Here's the drawing with two shaded views (mm, measured from the low corner). I have some questions. Coordinates: 2 decimals unless noted, no trailing zeros. Loops run counter-clockwise (first coordinate to the right, second up) from the corner with the lowest first, then second, coordinate; pieces in that order, holes last. Notation, with made-up numbers: (3.25, -8) -> (57.25, -8) arc R18 ccw to (57.25, 27) -> close; hole circle Ø11 at (79.25, 28.5). An arc over 180 degrees is marked (long way). Use CSV: the item, a comma, the result in double quotes. Start each with the question number.
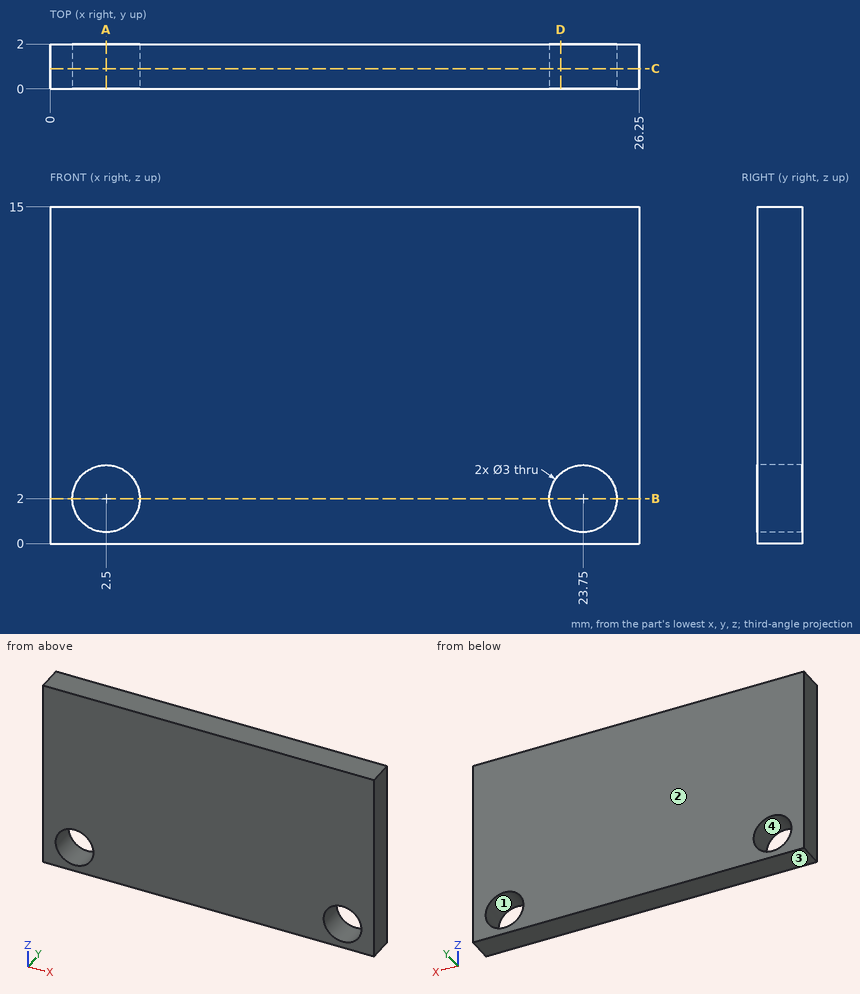
1) I want a section at B-B, the plane z = 2. Please give me the cut outline in (x, y).
2) Please list where these lines run through material, in increasing order: L1, parallel to X at y = 1.05, z = 2; L2, parallel to Z at x = 2.5, y = 0.8; L3, parallel to X at y = 0.25, z = 2.5. Write a range as [from, to].
3) I want a section at C-C, the plane y = 0.9. Please give me the cut outline in (x, z).
4) I want a section at D-D, the plane x = 22.75. Please give me the cut outline in (y, z), plus the area to 3 significant figures.
5) Thinking about a two-plate mould opening in Z: for the marked faces 1, 2, 3 and 4, which applies, pulls with the +Z half, pulls with the -Z half, needs draft (parallel to the pull), parting line crosses it, or undercut?
6) I want a section at A-A, the plane x = 2.5. Please give me the cut outline in (y, z).
7) For P1, Ø3.5, axis at x = 2.5, z = 2, coming from the -Y side, with a flat end and sliding along its axis, tell me the tip position at first contact or that it passes through.
Return value:
1,outline,"(0, 0) -> (1, 0) -> (1, 2) -> (0, 2) -> close; (4, 0) -> (22.25, 0) -> (22.25, 2) -> (4, 2) -> close; (25.25, 0) -> (26.25, 0) -> (26.25, 2) -> (25.25, 2) -> close"
2,L1,"x = [0, 1], [4, 22.25], [25.25, 26.25]"
2,L2,"z = [0, 0.5], [3.5, 15]"
2,L3,"x = [0, 1.09], [3.91, 22.34], [25.16, 26.25]"
3,outline,"(0, 0) -> (26.25, 0) -> (26.25, 15) -> (0, 15) -> close; hole circle Ø3 at (2.5, 2); hole circle Ø3 at (23.75, 2)"
4,outline,"(0, 0) -> (2, 0) -> (2, 0.88) -> (0, 0.88) -> close; (0, 3.12) -> (2, 3.12) -> (2, 15) -> (0, 15) -> close"
4,area,"25.5 mm²"
5,face 1,"undercut"
5,face 2,"needs draft"
5,face 3,"pulls with the -Z half"
5,face 4,"undercut"
6,outline,"(0, 0) -> (2, 0) -> (2, 0.5) -> (0, 0.5) -> close; (0, 3.5) -> (2, 3.5) -> (2, 15) -> (0, 15) -> close"
7,P1,"stops at y = 0"
